Source: CAD feature listing. Evaluate the final solid. Frame: model axes, mm. Face numbers are marked on the shaded views. A direction names the side the tool comes from. Give positions to 0.01 mm unless a question says otherwise; leave off trailing zeros. Order: outer loops, then holes, each group sorted by start corner. A loop starts at its lowest first (then second) coordinate and runs counter-clockwise, first axis right, second up.
```python
from build123d import *

# Parameters (mm, degrees)
SKETCH_R     = 2.1
PAD_DEPTH    = 1
SKETCH001_R  = 14
PAD001_DEPTH = 18
POCKET_DEPTH = 6
PAD002_DEPTH = 17
PAD003_DEPTH = 30


with BuildPart() as part:
    # Sketch → Pad (new body)
    with BuildSketch(Plane.XY):
        with BuildLine():
            ThreePointArc((13.555442, 3.5), (0, 14), (-13.555442, 3.5))
            Line((-17.5, 3.5), (-13.555442, 3.5))
            ThreePointArc((-17.5, 3.5), (-21, 0), (-17.5, -3.5))
            Line((-17.5, -3.5), (-13.555442, -3.5))
            ThreePointArc((-13.555442, -3.5), (0, -14), (13.555442, -3.5))
            Line((13.555442, -3.5), (17.5, -3.5))
            ThreePointArc((17.5, -3.5), (21, 0), (17.5, 3.5))
            Line((13.555442, 3.5), (17.5, 3.5))
        make_face()
        with Locations((-17.5, 0)):
            Circle(SKETCH_R, mode=Mode.SUBTRACT)
        with Locations((17.5, 0)):
            Circle(SKETCH_R, mode=Mode.SUBTRACT)
    extrude(amount=-PAD_DEPTH)

    # Sketch001 (on Face12 of Pad) → Pad001 (join)
    with BuildSketch(Plane(origin=(0, 0, -1), x_dir=(1, 0, 0), z_dir=(0, 0, -1))):
        Circle(SKETCH001_R)
    extrude(amount=PAD001_DEPTH)

    # Sketch002 → Revolution (revolve)
    with BuildSketch(Plane.XZ.offset(-8)):
        Polygon((0, 0), (4.5, 0), (4.5, 1.5), (2.5, 1.5), (2.5, 9.2), (1.7, 10), (0, 10), align=None)
    revolve(axis=Axis((0, 8, 0), (0, 0, 1)))

    # Sketch003 (on Face20 of Revolution) → Pocket (cut)
    with BuildSketch(Plane.XY.offset(10)):
        with BuildLine():
            ThreePointArc((2.598076, 9.5), (0, 11), (-2.598076, 9.5))
            Line((-2.598076, 9.5), (2.598076, 9.5))
        make_face()
        with BuildLine():
            Line((2.598076, 6.5), (-2.598076, 6.5))
            ThreePointArc((-2.598076, 6.5), (0, 5), (2.598076, 6.5))
        make_face()
    extrude(amount=-POCKET_DEPTH, mode=Mode.SUBTRACT)

    # Sketch004 → Pad002 (join)
    with BuildSketch(Plane.XY):
        with BuildLine():
            ThreePointArc((-7.3, -11.946129), (0, -14), (7.3, -11.946129))
            Line((7.3, -11.946129), (7.3, -17))
            Line((7.3, -17), (-7.3, -17))
            Line((-7.3, -17), (-7.3, -11.946129))
        make_face()
    extrude(amount=-PAD002_DEPTH)

    # Sketch005 (on Face22 of Pad002) → Pad003 (join)
    with BuildSketch(Plane.XZ.offset(17)):
        with BuildLine():
            ThreePointArc((-6.8, -0.5), (-7.3, -1), (-6.8, -1.5))
            Line((-6.8, -1.5), (6.8, -1.5))
            ThreePointArc((6.8, -1.5), (7.3, -1), (6.8, -0.5))
            Line((-6.8, -0.5), (6.8, -0.5))
        make_face()
    extrude(amount=PAD003_DEPTH)


solid = part.part
```
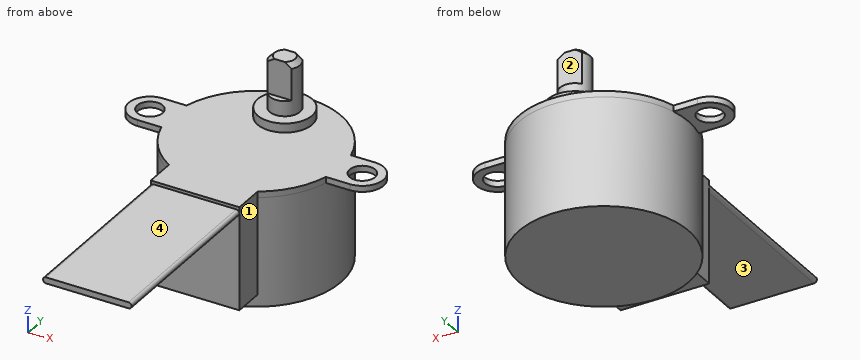
1) Reachability of the marked faces 1, 2, 3 and 4 from +Z, -Z, +X, -X, +Y, -Y: full face, straight path, thin tool, end or side. Return the list, or none.
Report:
face 1: +Z, -Z, +X, -Y
face 2: +Z, +X, -X, +Y
face 3: -Z, +X, -X, -Y
face 4: +Z, +X, -X, -Y
2) Material intervals for L1, parallel to Y at x = 17.5, z = -0.55; L2, parallel to Z at x = -3.5, y = -44; L3, parallel to Z at x = 6, y = -5, sorted ascending.
Report:
L1: y = -3.5 to -2.1, 2.1 to 3.5
L2: z = -1.5 to -0.5
L3: z = -19 to 0
3) Section query D-D, the plane y = -27. Return the cut outline in (x, z), and give its area (3 significant figures).
Report:
outline: (-6.8, -1.5) - (6.8, -1.5) arc R0.5 ccw to (6.8, -0.5) - (-6.8, -0.5) arc R0.5 ccw to start
area: 14.4 mm2
4) Section query C-C, the plane z = -6. Return the cut outline in (x, y).
Report:
outline: (-7.3, -17) - (7.3, -17) - (7.3, -11.95) arc R14 ccw (long way) to (-7.3, -11.95) - close
5) Pin query (flat end, axial travel): pin 1 (0.5 mm diameter, centred on x = 1, y = 10, fed in from +Z); pin 2 (15.5 mm diameter, centred on x = 5, y = -1.5, fed in from +Z); pin 3 (1.5 mm diameter, centred on y = -14.5, z = -8, fed in from -X); pin 4 (4 mm diameter, centred on x = -17.5, y = 0, fed in from -Z). Return the tip coordinate at first contact, or that it passes through.
Report:
pin 1: stops at z = 4
pin 2: stops at z = 1.5
pin 3: stops at x = -7.3
pin 4: passes through
6) Section query A-A, the plane y = 0. Return the cut outline in (x, z).
Report:
outline: (-21, -1) - (-19.6, -1) - (-19.6, 0) - (-21, 0) - close; (-15.4, -1) - (-14, -1) - (-14, -19) - (14, -19) - (14, -1) - (15.4, -1) - (15.4, 0) - (-15.4, 0) - close; (19.6, -1) - (21, -1) - (21, 0) - (19.6, 0) - close
7) Section query B-B, the plane x = 0. Return the cut outline in (y, z), and give its area (3 significant figures).
Report:
outline: (-47, -1.5) - (-17, -1.5) - (-17, -17) - (-14, -17) - (-14, -19) - (14, -19) - (14, 0) - (12.5, 0) - (12.5, 1.5) - (10.5, 1.5) - (10.5, 4) - (9.5, 4) - (9.5, 10) - (6.5, 10) - (6.5, 4) - (5.5, 4) - (5.5, 1.5) - (3.5, 1.5) - (3.5, 0) - (-17, 0) - (-17, -0.5) - (-47, -0.5) - close
area: 657 mm2
